```python
from build123d import *

# Parameters (mm, degrees)
F1_DEPTH = 5


# Not quite as in the source:
# - the program builds the solid bodies; features that only make, move or delete a surface that nothing else refers to are left out


with BuildPart() as f1:
    # F0 (on Front) → F1 (new body)
    with BuildSketch(Plane.XZ):
        with BuildLine():
            ThreePointArc((-38.5628677204, -8.4046955637), (-42.950748766, -19.8978357544), (-53.8815692168, -25.542562124))
            Line((-53.8815692168, -25.542562124), (-41.5648788357, -25.542562124))
            ThreePointArc((-41.5648788357, -25.542562124), (-35.6343803196, -17.869848935), (-33.5243537826, -8.4046955637))
            ThreePointArc((-33.5243537826, -8.4046955637), (-35.6391308825, 1.0705767284), (-41.5820798093, 8.7474527367))
            Line((-41.5820798093, 8.7474527367), (-54.0131150031, 8.7474527367))
            ThreePointArc((-54.0131150031, 8.7474527367), (-42.9949338553, 3.137686474), (-38.5628677204, -8.4046955637))
        make_face()
        with BuildLine():
            Line((-41.5648788357, -25.542562124), (-53.8815692168, -25.542562124))
            ThreePointArc((-53.8815692168, -25.542562124), (-73.0545080153, -8.4708549583), (-54.0131150031, 8.7474527367))
            Line((-54.0131150031, 8.7474527367), (-41.5820798093, 8.7474527367))
            ThreePointArc((-41.5820798093, 8.7474527367), (-78.0931460515, -8.4158741323), (-41.5648788357, -25.542562124))
        make_face()
        with BuildLine():
            ThreePointArc((-33.5243537826, -8.4046955637), (-35.6343803196, -17.869848935), (-41.5648788357, -25.542562124))
            Line((-41.5648788357, -25.542562124), (37.9639441457, -25.542562124))
            ThreePointArc((37.9639441457, -25.542562124), (55.1089515761, -8.3975546937), (37.9639441457, 8.7474527367))
            Line((37.9639441457, 8.7474527367), (-41.5820798093, 8.7474527367))
            ThreePointArc((-41.5820798093, 8.7474527367), (-35.6391308825, 1.0705767284), (-33.5243537826, -8.4046955637))
        make_face()
        with BuildLine():
            Line((37.9639441457, -20.3371653928), (37.9639441457, -17.8371653928))
            ThreePointArc((37.9639441457, -17.8371653928), (44.7629027111, -8.9185826964), (37.9639441457, 0))
            Line((37.9639441457, 0), (37.9639441457, 2.5))
            ThreePointArc((37.9639441457, 2.5), (48.2332452633, -8.9185826964), (37.9639441457, -20.3371653928))
        make_face(mode=Mode.SUBTRACT)
        with BuildLine():
            ThreePointArc((37.9639441457, 0), (44.7629027111, -8.9185826964), (37.9639441457, -17.8371653928))
            Line((37.9639441457, -17.8371653928), (37.9639441457, -20.3371653928))
            ThreePointArc((37.9639441457, -20.3371653928), (48.2332452633, -8.9185826964), (37.9639441457, 2.5))
            Line((37.9639441457, 2.5), (37.9639441457, 0))
        make_face()
    extrude(amount=F1_DEPTH)


solid = f1.part
```
Model file for the job. Use its own axes, mm. A direction names the side the tool comes from. Coordinates: 2 decimals unless noted, no trailing zeros. Loops run counter-clockwise (first coordinate to the right, second up) from the corner with the lowest first, then second, coordinate; pieces in that order, holes last. Notation, with made-up numbers: (65, -10.5) - (105, -10.5) arc R25 ccw to (105, 1.5) - close; hole circle Ø3 at (-29, 62). An arc over 180 degrees is marked (long way). Write item = value, one per line. Start each with the question number.
Item 1: Saw through at D-D, the plane x = -11. List the corners of the cut face in (y, z).
Item 2: Saw through at B-B, the plane z = -0.5. List the corners of the cut face in (x, y), then the cut area to 3 significant figures.
Item 3: Wall check: probe 1 along X at (y, z) = (-3.4, -9); probe 2 along Z at (x, y) = (16, -2.85); probe 3 along X at (y, z) = (-2.25, -5.5). Give the ranges that are in metal, low to high. Write a range as [from, to].
Item 4: Drop flat-ended pins along their axis: pin 1 Ø1 at (x, y) = (-44, -3) entering from +Z; pin 2 Ø2 at (x, y) = (-18.5, -4) entering from -Z; pin 3 Ø1.5 at (y, z) = (-4, 4.5) entering from -X. Give the stop position or say it passes through.
Item 5: 3-axis set-ups, long thin cutter, end or side, ignore diameter. For faces 1 (the face through (-1, -2, 8.747)), 2 (the face through (2, 0, -8)), 3 (the face through (-2, -2, -25.543)): which of +Z, -Z, +X, -X, +Y, -Y reach the whole face in a straight line?
Item 6: Saw through at A-A, the plane y = -4. List the corners of the cut face in (x, z) (3 decimals).
Item 7: Saw through at C-C, the plane x = -66. List the corners of the cut face in (y, z), then the cut area to 3 significant figures.
Answers:
q1.outline = (-5, -25.54) - (0, -25.54) - (0, 8.75) - (-5, 8.75) - close
q2.outline = (-76.64, -5) - (-71.14, -5) - (-71.14, 0) - (-76.64, 0) - close; (-40.48, -5) - (53.18, -5) - (53.18, 0) - (-40.48, 0) - close
q2.area = 496 mm2
q3.probe_1 = [-78.09, -73.04], [-38.57, 55.1]
q3.probe_2 = [-25.54, 8.75]
q3.probe_3 = [-77.9, -72.81], [-38.81, 54.86]
q4.pin_1 = 10.8
q4.pin_2 = -25.54
q4.pin_3 = -74.49
q5.face_1 = +Z, +X, +Y, -Y
q5.face_2 = +Z, -Z, +X, -X, +Y
q5.face_3 = -Z, +X, +Y, -Y
q6.outline = (-41.582, 8.747) arc R22.284 ccw (long way) to (-41.565, -25.543) - (37.964, -25.543) arc R17.145 ccw to (37.964, 8.747) - close; hole circle Ø34.492 at (-55.809, -8.405)
q7.outline = (-5, -28.22) - (0, -28.22) - (0, -22.32) - (-5, -22.32) - close; (-5, 5.51) - (0, 5.51) - (0, 11.41) - (-5, 11.41) - close
q7.area = 59.0 mm2
